Answer from the drawing. Dimensions are ordinates in mm from the lowest x, y and z of the part. A direction names the side the tool comes from. Round coordinates to 2 decimals unless told otherwise and drop trailing zeros. Write each loop counter-clockwise with the first axis right and the second up, starting at its lowest first coordinate (ties: lowest second). Pieces come first, ordered by that corner, then holes. Notation, with made-up numbers: (49, 47) - (74, 47) arc R16 cw to (74, 64) - close; hole circle Ø9 at (35, 30). An arc over 180 degrees is marked (long way). Use a Markdown table: item, result. Add a question column.
1) A cutting plane is placed at B-B (x = 64.67). Give the vertices of the cut face in (y, z).
2) A cutting plane is placed at C-C (y = 2.5). Give the vertices of the cut face in (x, z), then the cut area to 3 significant figures.
3) A cutting plane is placed at A-A (z = 6.35). Give the vertices of the cut face in (x, y), then the cut area to 3 significant figures.
4) A tool of negligible diameter and unlimited length cuts with its end or side. For the marked faces 4, 5 and 6, from which of +Z, -Z, +X, -X, +Y, -Y can it reach the whole face along a straight path? Write none if from no direction.
5) A cutting plane is placed at D-D (y = 12.5). Give the vertices of the cut face in (x, z).
6) Each of these flat-tipped pins is pushed along its axis until it touches: P1, Ø5, axis at x = 46, y = 10, coming from the -Z side; P2, Ø4, axis at y = 21, z = 11.5, coming from the +X side; P3, Ø4, axis at x = 29, z = 11.5, coming from the +Y side; P4, Ø3, axis at x = 63.5, z = 9, coming from the +Y side. Where does it stop, or does it pass through?
7) Determine the mould class of the marked faces 1, 2 and 3 for opening direction X: +X half, -X half, draft (parallel to the pull), parting line (faces both ways), or undercut.
8) Find the intervals of material crossed by probe 1 along X at (y, z) = (1.6, 6.35); probe 2 along X at (y, z) = (3.3, 6.35); probe 3 along Y at (x, z) = (59.5, 11.75), in increasing order. Write a range as from..to.
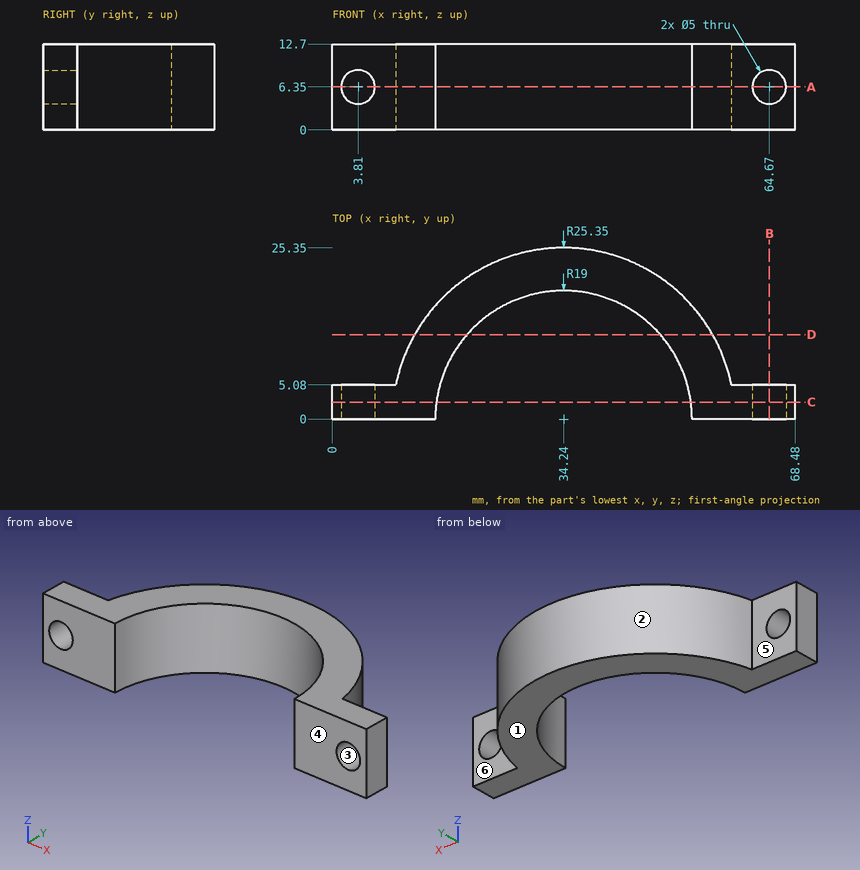
Entries:
| question | item | result |
|---|---|---|
| 1 | outline | (0, 0) - (5.08, 0) - (5.08, 3.85) - (0, 3.85) - close; (0, 8.85) - (5.08, 8.85) - (5.08, 12.7) - (0, 12.7) - close |
| 2 | outline | (0, 0) - (15.41, 0) - (15.41, 12.7) - (0, 12.7) - close; (53.07, 0) - (68.48, 0) - (68.48, 12.7) - (53.07, 12.7) - close; hole circle Ø5 at (3.81, 6.35); hole circle Ø5 at (64.67, 6.35) |
| 2 | area | 352 mm² |
| 3 | outline | (0, 0) - (1.31, 0) - (1.31, 5.08) - (0, 5.08) - close; (6.31, 0) - (15.24, 0) arc R19 cw to (53.24, 0) - (62.17, 0) - (62.17, 5.08) - (59.08, 5.08) arc R25.35 ccw to (9.4, 5.08) - (6.31, 5.08) - close; (67.17, 0) - (68.48, 0) - (68.48, 5.08) - (67.17, 5.08) - close |
| 3 | area | 484 mm² |
| 4 | face 4 | +Z, -Z, +X, -X, -Y |
| 4 | face 5 | +Z, -Z, -X, +Y |
| 4 | face 6 | +Z, -Z, +X, +Y |
| 5 | outline | (12.19, 0) - (19.93, 0) - (19.93, 12.7) - (12.19, 12.7) - close; (48.55, 0) - (56.29, 0) - (56.29, 12.7) - (48.55, 12.7) - close |
| 6 | P1 | passes through |
| 6 | P2 | stops at x = 51.02 |
| 6 | P3 | stops at y = 25.14 |
| 6 | P4 | stops at y = 5.08 |
| 7 | face 1 | draft |
| 7 | face 2 | parting line |
| 7 | face 3 | undercut |
| 8 | probe 1 | x = 0..1.31, 6.31..15.31, 53.17..62.17, 67.17..68.48 |
| 8 | probe 2 | x = 0..1.31, 6.31..15.53, 52.95..62.17, 67.17..68.48 |
| 8 | probe 3 | y = 0..5.08 |
